Here's how the part is built. I have some questions about the finished solid (model axes, mm). Coordinates: 2 decimals unless noted, no trailing zeros. Loops run counter-clockwise (first coordinate to the right, second up) from the corner with the lowest first, then second, coordinate; pieces in that order, holes last. Notation, with made-up numbers: M 53,83.25 L 73,83.25 A31 cw 73,120.25 Z; hole C 5,-12 d10. An arc over 180 degrees is marked long. Use one line per item in the form item = value. Start each with the question number.
(1) Imagine slicing it at B-B, the plane z = 91. Please give me the cut outline in (x, y).
(2) Will these pins go through, and if not, where does the flat tip stop? P1, Ø2, axis at x = -23.5, y = 2, coming from the -Z side; P2, Ø1.2, axis at y = 2, z = 93.5, coming from the -X side; P3, Ø2, axis at y = 2, z = -24.5, coming from the +X side.
(3) Please list where these lines run through material, in increasing order: L1, parallel to X at y = 3.2, z = 6; L2, parallel to Z at x = -103, y = 2.45; L3, parallel to Z at x = 36, y = 0.95.
(4) Imagine slicing it at D-D, the plane x = -20.5. Please give me the cut outline in (y, z), and give its area (3 significant figures).
(5) Imagine slicing it at A-A, the plane z = -25. Please give me the cut outline in (x, y), and give its area (3 significant figures).
(6) Imagine slicing it at C-C, the plane z = 42. Please give me the cut outline in (x, y), and give its area (3 significant figures).
(7) Thinking about a two-plate mould opening in X: for faces 1 (the cylindrical face through (34.11, 1.97, -46.35)), 2 (the cylindrical face through (-140.61, 1.97, -54.52)), 3 (the cylindrical face through (52.736, 1.972, 117.43)), which applies, +X half, -X half, draft (parallel to the pull), parting line (faces both ways), or undercut?
```python
from build123d import *

# Parameters (mm, degrees)
SKETCH1_R           = 20
SKETCH1_R_2         = 2.32
SKETCH1_R_3         = 2
SKETCH1_W           = 10
SKETCH1_H           = 60
SKETCH1_W_2         = 15
SKETCH1_H_2         = 25
BOSS_EXTRUDE1_DEPTH = 4
FILLET2_R           = 20
FILLET3_R           = 25


with BuildPart() as part:
    # Sketch1 → Boss-Extrude1 (new body)
    with BuildSketch(Plane(origin=(0, 0, 0), x_dir=(1, 0, 0), z_dir=(0, 1, 0))):
        Polygon((-150, 43.493460664), (-114, 43.493460664), (-114, -106.506539336), (-150, -106.506539336), (-150, -121.506539336), (60, -121.506539336), (60, -106.506539336), (24, -106.506539336), (24, 43.493460664), (60, 43.493460664), (60, 58.493460664), (0, 58.493460664), (0, -3.506539336), (-90, -3.506539336), (-90, 58.493460664), (-150, 58.493460664), align=None)
        with Locations(Location((-45.147898231, -31.506539336, 0), (0, 0, 270))):
            Circle(SKETCH1_R, mode=Mode.SUBTRACT)
        with Locations(Location((-125, -111.506539336, 0), (0, 0, 270))):
            Circle(SKETCH1_R_2, mode=Mode.SUBTRACT)
        with Locations(Location((-125, 48.493460664, 0), (0, 0, 90))):
            Circle(SKETCH1_R_2, mode=Mode.SUBTRACT)
        with Locations(Location((35, 48.493460664, 0), (0, 0, 270))):
            Circle(SKETCH1_R_2, mode=Mode.SUBTRACT)
        with Locations(Location((35, -111.506539336, 0), (0, 0, 90))):
            Circle(SKETCH1_R_2, mode=Mode.SUBTRACT)
        with Locations(Location((-85, -96.506539336, 0), (0, 0, 270))):
            Circle(SKETCH1_R_3, mode=Mode.SUBTRACT)
        with Locations(Location((-5, -96.506539336, 0), (0, 0, 90))):
            Circle(SKETCH1_R_3, mode=Mode.SUBTRACT)
        with Locations(Location((-85, -16.506539336, 0), (0, 0, 90))):
            Circle(SKETCH1_R_3, mode=Mode.SUBTRACT)
        with Locations(Location((-5, -16.506539336, 0), (0, 0, 270))):
            Circle(SKETCH1_R_3, mode=Mode.SUBTRACT)
        with Locations((13, -31.506539336)):
            Rectangle(SKETCH1_W, SKETCH1_H, mode=Mode.SUBTRACT)
        with Locations((-103, -31.506539336)):
            Rectangle(SKETCH1_W, SKETCH1_H, mode=Mode.SUBTRACT)
        with Locations((10.5, -99.006539336)):
            Rectangle(SKETCH1_W_2, SKETCH1_H_2, mode=Mode.SUBTRACT)
        with Locations((-100.5, -99.006539336)):
            Rectangle(SKETCH1_W_2, SKETCH1_H_2, mode=Mode.SUBTRACT)
    extrude(amount=BOSS_EXTRUDE1_DEPTH)

    # Fillet2
    # the kernel refuses this fillet: 20 mm, written as the material it takes off along each edge
    with BuildSketch(Plane(origin=(60, -48.412291828, 121.506539336), x_dir=(-1, 0, 0), z_dir=(0, 1, 0))) as fillet2_piece_1:
        with BuildLine():
            CenterArc((19.364916731, -20), FILLET2_R, 90, 75.522487814)
            Line((0, -15), (-0.387298335, -14.9))
            ThreePointArc((-0.387298335, -14.9), (-0.4, -7.5), (-0.4, 0))
            Line((-0.4, 0), (0, 0.4))
            Line((0, 0.4), (19.364916731, 0.4))
            Line((19.364916731, 0.4), (19.364916731, 0))
        make_face()
    extrude(amount=100.824583655, mode=Mode.SUBTRACT)
    with BuildSketch(Plane(origin=(-150, -48.412291828, 121.506539336), x_dir=(0, 0, -1), z_dir=(0, 1, 0))) as fillet2_piece_2:
        with BuildLine():
            CenterArc((20, -19.364916731), FILLET2_R, 104.477512186, 75.522487814)
            Line((0, -19.364916731), (-0.4, -19.364916731))
            Line((-0.4, -19.364916731), (-0.4, 0))
            Line((-0.4, 0), (0, 0.4))
            ThreePointArc((0, 0.4), (7.5, 0.4), (14.9, 0.387298335))
            Line((14.9, 0.387298335), (15, 0))
        make_face()
    extrude(amount=100.824583655, mode=Mode.SUBTRACT)

    # Fillet3
    # the kernel refuses this fillet: 25 mm, written as the material it takes off along each edge
    with BuildSketch(Plane(origin=(60, -57.282196187, -58.493460664), x_dir=(-1, 0, 0), z_dir=(0, 1, 0))) as fillet3_piece_1:
        with BuildLine():
            CenterArc((22.912878475, 25), FILLET3_R, 203.578178478, 66.421821522)
            Line((0, 15), (-0.458257569, 14.8))
            ThreePointArc((-0.458257569, 14.8), (-0.5, 7.5), (-0.5, 0))
            Line((-0.5, 0), (0, -0.5))
            Line((0, -0.5), (22.912878475, -0.5))
            Line((22.912878475, -0.5), (22.912878475, 0))
        make_face()
    extrude(amount=118.564392374, mode=Mode.SUBTRACT)
    with BuildSketch(Plane(origin=(-150, -57.282196187, -58.493460664), x_dir=(0, 0, 1), z_dir=(0, 1, 0))) as fillet3_piece_2:
        with BuildLine():
            CenterArc((25, 22.912878475), FILLET3_R, 180, 66.421821522)
            Line((0, 22.912878475), (-0.5, 22.912878475))
            Line((-0.5, 22.912878475), (-0.5, 0))
            Line((-0.5, 0), (0, -0.5))
            ThreePointArc((0, -0.5), (7.5, -0.5), (14.8, -0.458257569))
            Line((14.8, -0.458257569), (15, 0))
        make_face()
    extrude(amount=118.564392374, mode=Mode.SUBTRACT)


solid = part.part
```
Answer:
q1.outline = M -114,0 L -108,0 L -108,4 L -114,4 Z; M -93,0 L 3,0 L 3,4 L -93,4 Z; M 18,0 L 24,0 L 24,4 L 18,4 Z
q2.P1 = 3.51
q2.P2 = -114
q2.P3 = 24
q3.L1 = -114 to -108, -98 to 8, 18 to 24
q3.L2 = -58.49 to 1.51, 61.51 to 86.51, 111.51 to 121.51
q3.L3 = -58.49 to -50.59, -46.4 to -43.49, 106.51 to 109.41, 113.6 to 121.51
q4.outline = M 0,3.51 L 4,3.51 L 4,121.51 L 0,121.51 Z
q4.area = 472 mm²
q5.outline = M -114,0 L -90,0 L -90,4 L -114,4 Z; M 0,0 L 24,0 L 24,4 L 0,4 Z
q5.area = 192 mm²
q6.outline = M -114,0 L -108,0 L -108,4 L -114,4 Z; M -98,0 L -62.17,0 L -62.17,4 L -98,4 Z; M -28.12,0 L 8,0 L 8,4 L -28.12,4 Z; M 18,0 L 24,0 L 24,4 L 18,4 Z
q6.area = 336 mm²
q7.face_1 = undercut
q7.face_2 = -X half
q7.face_3 = +X half
